The listing builds one solid part. Answer for the finished solid, in the listing's coordinates (mm). Face numbers are marked on the shaded views. Round coordinates to 2 decimals unless told otherwise and drop trailing zeros. Loops run counter-clockwise (first coordinate to the right, second up) from the corner with the lowest first, then second, coordinate; pieces in that order, holes last. Notation, with made-up numbers: (25.25, 36) - (51.25, 36) arc R21 cw to (51.25, 46) - close; hole circle Ø4 at (24.5, 33.25). An arc over 180 degrees is marked (long way). One line per item, written item: value.
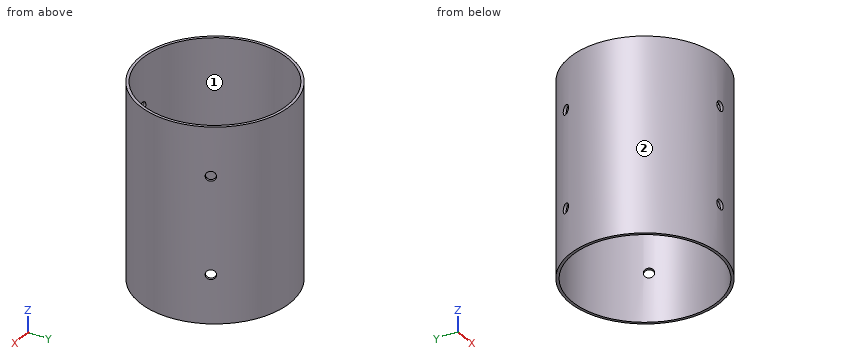
```python
from build123d import *

# Parameters (mm, degrees)
SKETCH1_R           = 49.5046
SKETCH1_R_2         = 47.6885
BOSS_EXTRUDE1_DEPTH = 127
SKETCH4_R           = 3.175
CUT_EXTRUDE3_DEPTH  = 50.5046
CIRPATTERN2_COUNT   = 3


with BuildPart() as part:
    # Sketch1 → Boss-Extrude1 (new body)
    with BuildSketch(Plane.XY):
        Circle(SKETCH1_R)
        Circle(SKETCH1_R_2, mode=Mode.SUBTRACT)
    extrude(amount=BOSS_EXTRUDE1_DEPTH)

    # Sketch4 → Cut-Extrude3 (cut, through all)
    with BuildSketch(Plane(origin=(0, 0, 0), x_dir=(1, 0, 0), z_dir=(0, 1, 0))):
        with Locations((0, -31.75)):
            Circle(SKETCH4_R)
        with Locations((0, -95.25)):
            Circle(SKETCH4_R)
    cut_extrude3 = extrude(amount=-CUT_EXTRUDE3_DEPTH, mode=Mode.SUBTRACT)

    # CirPattern2: Cut-Extrude3 ×3 about axis
    cirpattern2_axis = Axis((0, 0, 127), (0, 0, -1))
    for i in range(1, CIRPATTERN2_COUNT):
        add(cut_extrude3.rotate(cirpattern2_axis, i * 360 / CIRPATTERN2_COUNT), mode=Mode.SUBTRACT)


solid = part.part
```
1) A cutting plane is placed at A-A on x = 0. Give the vertices of the cut face in (y, z) (1 decimal), and give its area (3 significant figures).
Final values:
outline: (-49.5, 0) - (-47.7, 0) - (-47.7, 28.6) - (-49.5, 28.6) - close; (-49.5, 34.9) - (-47.7, 34.9) - (-47.7, 92.1) - (-49.5, 92.1) - close; (-49.5, 98.4) - (-47.7, 98.4) - (-47.7, 127) - (-49.5, 127) - close; (47.7, 0) - (49.5, 0) - (49.5, 127) - (47.7, 127) - close
area: 438 mm2
2) Consider L1, parallel to Z at x = 0, y = -48.05 (3 decimals); L2, parallel to X at y = -0.5, z = 16.5; L3, parallel to X at y = 26.5, z = 29. Determine where each line is inside the solid, lowest interval first.
Final values:
L1: 0 to 28.575, 34.925 to 92.075, 98.425 to 127
L2: -49.5 to -47.69, 47.69 to 49.5
L3: -41.81 to -39.65, 39.65 to 41.81
3) For a pull along Y with two mould halves and no side action, classify the marked faces 1 and 2 as released by +Y, released by -Y, zero draft, split by the parting line, or undercut.
Final values:
face 1: undercut
face 2: split by the parting line
4) A cutting plane is placed at B-B on y = 0. Give the vertices of the cut face in (x, z).
Final values:
outline: (-49.5, 0) - (-47.69, 0) - (-47.69, 127) - (-49.5, 127) - close; (47.69, 0) - (49.5, 0) - (49.5, 127) - (47.69, 127) - close
5) Each of these flat-tipped pins is pushed along its axis until it touches: pin 1 Ø12 at (x, z) = (26.5, 107.5) entering from +Y; pin 2 Ø12 at (y, z) = (-10, 40.5) entering from -X; pin 3 Ø8 at (y, z) = (37.5, 43) entering from -X. Where does it stop, or does it pass through?
Final values:
pin 1: y = 45.06
pin 2: x = -49.34
pin 3: x = -36.45
6) A cutting plane is placed at C-C on x = 32. Give the vertices of the cut face in (y, z), and give its area (3 significant figures).
Final values:
outline: (-37.77, 0) - (-35.36, 0) - (-35.36, 127) - (-37.77, 127) - close; (35.36, 0) - (37.77, 0) - (37.77, 127) - (35.36, 127) - close
area: 613 mm2
7) A cutting plane is placed at D-D on z = 31.75. Give the vertices of the cut face in (x, y) (1 decimal).
Final values:
outline: (-44.4, 22) arc R49.5 ccw to (-3.2, -49.4) - (-3.2, -47.6) arc R47.7 cw to (-42.8, 21) - close; (-41.2, 27.5) - (-39.6, 26.5) arc R47.7 cw to (39.6, 26.5) - (41.2, 27.5) arc R49.5 ccw to start; (3.2, -49.4) arc R49.5 ccw to (44.4, 22) - (42.8, 21) arc R47.7 cw to (3.2, -47.6) - close
